```python
from build123d import *

# Parameters (mm, degrees)
BOX_W           = 36
BOX_H           = 36
BOX_DEPTH       = 36
SKETCH_R        = 3
POCKET_DEPTH    = 2
SKETCH001_R     = 3
POCKET001_DEPTH = 2
SKETCH002_R     = 3
POCKET002_DEPTH = 2
SKETCH003_R     = 3
POCKET003_DEPTH = 2
SKETCH004_R     = 3
POCKET004_DEPTH = 2
SKETCH005_R     = 3
POCKET005_DEPTH = 2


with BuildPart() as sphere:
    # Sphere → Sphere (revolve)
    with BuildSketch(Plane.XZ):
        with BuildLine():
            ThreePointArc((0, -25), (25, 0), (0, 25))
            Line((0, 25), (0, -25))
        make_face()
    revolve(axis=Axis((0, 0, 0), (0, 0, 1)))


with BuildPart() as f_1_furo:
    # Box → Box (new body)
    with BuildSketch(Plane(origin=(-18, -18, -18), x_dir=(1, 0, 0), z_dir=(0, 0, 1))):
        with Locations((18, 18)):
            Rectangle(BOX_W, BOX_H)
    extrude(amount=BOX_DEPTH)

    # Common: intersect Sphere
    add(sphere.part, mode=Mode.INTERSECT)

    # Sketch → Pocket (cut)
    with BuildSketch(Plane.YZ.offset(18)):
        with Locations((-8, 8)):
            Circle(SKETCH_R)
        with Locations((-8, -8)):
            Circle(SKETCH_R)
        with Locations((8, 8)):
            Circle(SKETCH_R)
        with Locations((8, -8)):
            Circle(SKETCH_R)
        with Locations((-8, 0)):
            Circle(SKETCH_R)
        with Locations((8, 0)):
            Circle(SKETCH_R)
    extrude(amount=-POCKET_DEPTH, mode=Mode.SUBTRACT)

    # Sketch001 → Pocket001 (cut)
    with BuildSketch(Plane(origin=(0, 18, 0), x_dir=(-1, 0, 0), z_dir=(0, 1, 0))):
        with Locations((8, 8)):
            Circle(SKETCH001_R)
        with Locations((-8, 8)):
            Circle(SKETCH001_R)
        with Locations((-8, -8)):
            Circle(SKETCH001_R)
        with Locations((8, -8)):
            Circle(SKETCH001_R)
        Circle(SKETCH001_R)
    extrude(amount=-POCKET001_DEPTH, mode=Mode.SUBTRACT)

    # Sketch002 → Pocket002 (cut)
    with BuildSketch(Plane(origin=(-18, 0, 0), x_dir=(0, -1, 0), z_dir=(-1, 0, 0))):
        with Locations((-8, 8)):
            Circle(SKETCH002_R)
        with Locations((8, 8)):
            Circle(SKETCH002_R)
        with Locations((8, -8)):
            Circle(SKETCH002_R)
        with Locations((-8, -8)):
            Circle(SKETCH002_R)
    extrude(amount=-POCKET002_DEPTH, mode=Mode.SUBTRACT)

    # Sketch003 → Pocket003 (cut)
    with BuildSketch(Plane.XZ.offset(18)):
        with Locations((-8, 8)):
            Circle(SKETCH003_R)
        Circle(SKETCH003_R)
        with Locations((8, -8)):
            Circle(SKETCH003_R)
    extrude(amount=-POCKET003_DEPTH, mode=Mode.SUBTRACT)

    # Sketch004 → Pocket004 (cut)
    with BuildSketch(Plane(origin=(0, 0, -18), x_dir=(1, 0, 0), z_dir=(0, 0, -1))):
        with Locations((-8, 8)):
            Circle(SKETCH004_R)
        with Locations((8, -8)):
            Circle(SKETCH004_R)
    extrude(amount=-POCKET004_DEPTH, mode=Mode.SUBTRACT)

    # Sketch005 → Pocket005 (cut)
    with BuildSketch(Plane.XY.offset(18)):
        Circle(SKETCH005_R)
    extrude(amount=-POCKET005_DEPTH, mode=Mode.SUBTRACT)


solid = f_1_furo.part
```
Model file for the job. Use its own axes, mm. A direction names the side the tool comes from. Coordinates: 2 decimals unless noted, no trailing zeros. Write each loop counter-clockwise with the first axis right and the second up, starting at its lowest first coordinate (ties: lowest second). Pieces come first, ordered by that corner, then holes. Notation, with made-up numbers: (54.5, -37.5) - (89.5, -37.5) arc R26 ccw to (89.5, -3.5) - close; hole circle Ø8 at (37, 63.25). An arc over 180 degrees is marked (long way). Use a Markdown table: item, result. Add a question column.
Item 1: Drill centre lines: line 1 along Z through (x, y) = (17.1, -8); line 2 along Z through (x, y) = (-17.5, -8); line 3 along Y through (x, z) = (10.5, 9). Where is each one in solid material? Low to high.
Item 2: Band-saw the part on D-D, the plane z = -0.5. Write the cut outline in (x, y) (3 decimals).
Item 3: 3-axis set-ups, long thin cutter, end or side, ignore diameter. For faces 4 (the face through (5.14, 17.01, -7.1)), 5 (the face through (-17.01, -10.86, 8.9)), 6 (the face through (17.01, -5.14, -7.1)), 7 (the face through (-3, 0, 17)): which of +Z, -Z, +X, -X, +Y, -Y reach the whole face in a straight line?
Item 4: Two-plate mould, pull along X, no slides. Class faces 1 (the face through (16, -8, 8)), 2 (the face through (-16, 8, -8)), 3 (the face through (0, -16, 0)): pulls with the +X half, pulls with the -X half, needs draft (parallel to the pull), parting line crosses it, or undercut.
Item 5: Band-saw the part on A-A, the plane x = 0. Write the cut outline in (y, z), and give its area (3 significant figures).
Item 6: Band-saw the part on C-C, the plane z = 16.5. Write the cut outline in (x, y).
Item 7: Drop flat-ended pins along their axis: pin 1 (5 mm diameter, centred on y = 8, z = 8, fed in from +X); pin 2 (3 mm diameter, centred on x = -9, y = -9, fed in from -Z); pin 3 (3 mm diameter, centred on y = -7, z = 7, fed in from -X). Give the stop position or say it passes through.
A:
| question | item | result |
|---|---|---|
| 1 | line 1 | z = -16.39 to -11, -5 to -3, 3 to 5, 11 to 16.39 |
| 1 | line 2 | z = -15.96 to -11, -5 to 5, 11 to 15.96 |
| 1 | line 3 | y = -18 to 16 |
| 2 | outline | (-18, -17.342) arc R24.995 ccw to (-17.342, -18) - (-2.958, -18) - (-2.958, -16) - (2.958, -16) - (2.958, -18) - (17.342, -18) arc R24.995 ccw to (18, -17.342) - (18, -10.958) - (16, -10.958) - (16, -5.042) - (18, -5.042) - (18, 5.042) - (16, 5.042) - (16, 10.958) - (18, 10.958) - (18, 17.342) arc R24.995 ccw to (17.342, 18) - (2.958, 18) - (2.958, 16) - (-2.958, 16) - (-2.958, 18) - (-17.342, 18) arc R24.995 ccw to (-18, 17.342) - close |
| 3 | face 4 | +Y |
| 3 | face 5 | -X |
| 3 | face 6 | +X |
| 3 | face 7 | +Z |
| 4 | face 1 | pulls with the +X half |
| 4 | face 2 | pulls with the -X half |
| 4 | face 3 | undercut |
| 5 | outline | (-18, -17.35) arc R25 ccw to (-17.35, -18) - (17.35, -18) arc R25 ccw to (18, -17.35) - (18, -3) - (16, -3) - (16, 3) - (18, 3) - (18, 17.35) arc R25 ccw to (17.35, 18) - (3, 18) - (3, 16) - (-3, 16) - (-3, 18) - (-17.35, 18) arc R25 ccw to (-18, 17.35) - (-18, 3) - (-16, 3) - (-16, -3) - (-18, -3) - close |
| 5 | area | 1,260 mm² |
| 6 | outline | (-18, -5.36) arc R18.78 ccw to (-5.36, -18) - (5.36, -18) arc R18.78 ccw to (18, -5.36) - (18, 5.36) arc R18.78 ccw to (5.36, 18) - (-5.36, 18) arc R18.78 ccw to (-18, 5.36) - close; hole circle Ø6 at (0, 0) |
| 7 | pin 1 | stops at x = 16 |
| 7 | pin 2 | stops at z = -16 |
| 7 | pin 3 | stops at x = -16 |
